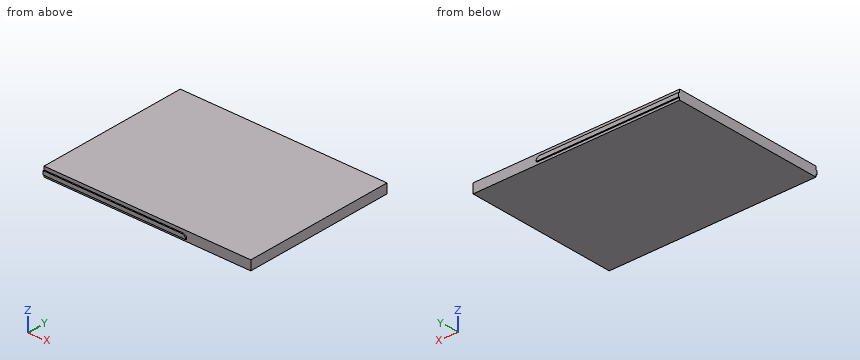
```python
from build123d import *

# Parameters (mm, degrees)
ESBO_O1_W                     = 217.3
ESBO_O1_H                     = 159.8
RESSALTO_EXTRUS_O1_DEPTH      = 10
RESSALTO_EXTRUS_O2_DEPTH      = 1.24
RESSALTO_EXTRUS_O2_DEPTH_BACK = 161.04
ESBO_O2_W                     = 150
ESBO_O2_H                     = 4
FILETE1_R                     = 4
FILETE2_R                     = 4


with BuildPart() as part:
    # Esboço1 → Ressalto-extrusão1 (new body)
    with BuildSketch(Plane.XY):
        with Locations((41.520834075, -42.82072758)):
            Rectangle(ESBO_O1_W, ESBO_O1_H)
    extrude(amount=RESSALTO_EXTRUS_O1_DEPTH)

    # Esboço2 → Ressalto-extrusão2 (add, two sides: drawn at the far end of the back side and taken through both)
    with BuildSketch(Plane(origin=(0, 37.07927242, 0), x_dir=(1, 0, 0), z_dir=(0, 1, 0)).offset(-RESSALTO_EXTRUS_O2_DEPTH_BACK)):
        with Locations((7.870834075, -4.5)):
            Rectangle(ESBO_O2_W, ESBO_O2_H)
    extrude(amount=RESSALTO_EXTRUS_O2_DEPTH + RESSALTO_EXTRUS_O2_DEPTH_BACK)

    # Filete1
    filete1_edges = [part.edges().sort_by_distance(p)[0] for p in [
        (82.870834075, -123.34072758, 6.5),
    ]]
    fillet(filete1_edges, radius=FILETE1_R - 0.0001)  # a hair under: the kernel refuses the full size

    # Filete2
    filete2_edges = [part.edges().sort_by_distance(p)[0] for p in [
        (82.870834075, 37.69927242, 6.5),
    ]]
    fillet(filete2_edges, radius=FILETE2_R - 0.0001)  # a hair under: the kernel refuses the full size


solid = part.part
```
Can you work these out from the model? Positions are in its coordinate system, mm. Round coordinates to 2 decimals unless told otherwise and drop trailing zeros. Loops run counter-clockwise (first coordinate to the right, second up) from the corner with the lowest first, then second, coordinate; pieces in that order, holes last. Notation, with made-up numbers: M 30.5,30.25 L 42.5,30.25 A28 ccw 42.5,52.25 Z; hole C -3.5,80 d10. An arc over 180 degrees is marked long. Answer as a JSON object with one key per item and string values. Group by question number.
Q1. Will these pins go through, and if not, where does the flat tip stop? pin 1 (1 mm diameter, centred on x = 22.5, z = 7.5, fed in from +Y); pin 2 (1.4 mm diameter, centred on x = 20, y = 38, fed in from -Z).
Q2. Please list where this line runs through material, in increasing order: L1, parallel to Y at x = 141.5, z = 1.
Q3. Imagine slicing it at B-B, the plane z = 8. Please give me the cut outline in (x, y), then the cut area to 3 significant figures.
Q4. Imagine slicing it at A-A, the plane x = 131. Please give me the cut outline in (y, z), then the cut area to 3 significant figures.
Findings:
{
 "1": {"pin 1": "stops at y = 37.08", "pin 2": "stops at z = 2.5"},
 "2": {"L1": "y = -122.72 to 37.08"},
 "3": {"outline": "M -67.13,-122.72 L 150.17,-122.72 L 150.17,37.08 L -67.13,37.08 Z", "area": "34,700 mm2"},
 "4": {"outline": "M -122.72,0 L 37.08,0 L 37.08,10 L -122.72,10 Z", "area": "1,600 mm2"}
}
